from build123d import *

# Parameters (mm, degrees)
BOSS_EXTRUDE1_DEPTH = 30.5
SKETCH4_W           = 23.4
SKETCH4_H           = 13
CUT_EXTRUDE2_DEPTH  = 25
CUT_EXTRUDE4_DEPTH  = 11.5
SKETCH7_W           = 31
SKETCH7_H           = 1.7
BOSS_EXTRUDE3_DEPTH = 6
BOSS_EXTRUDE4_DEPTH = 6
LPATTERN1_COUNT     = 10
LPATTERN1_PITCH     = 3.1
SKETCH11_W          = 12
SKETCH11_H          = 4.5
BOSS_EXTRUDE5_DEPTH = 3
FILLET1_R           = 2
FILLET2_R           = 2
FILLET5_R           = 3
SKETCH12_W          = 3.5
SKETCH12_H          = 3.5
CUT_EXTRUDE5_DEPTH  = 12
FILLET6_R           = 1.5


with BuildPart() as part:
    # Sketch1 → Boss-Extrude1 (new body)
    with BuildSketch(Plane.XY):
        Polygon((0, 0), (0, -30), (12, -30), (12, -20), (5, 0), align=None)
    extrude(amount=-BOSS_EXTRUDE1_DEPTH)

    # Sketch4 → Cut-Extrude2 (cut)
    with BuildSketch(Plane.ZY):
        with Locations((-14.5, -25.899949695)):
            Rectangle(SKETCH4_W, SKETCH4_H)
    extrude(amount=-CUT_EXTRUDE2_DEPTH, mode=Mode.SUBTRACT)

    # Sketch6 → Cut-Extrude4 (cut, symmetric)
    with BuildSketch(Plane.XY.offset(-15.25)):
        Polygon((5, 0), (5, -14), (9.9, -14), align=None)
    extrude(amount=CUT_EXTRUDE4_DEPTH, both=True, mode=Mode.SUBTRACT)

    # Sketch7 → Boss-Extrude3 (add)
    with BuildSketch(Plane(origin=(0, -28, 0), x_dir=(1, 0, 0), z_dir=(0, 1, 0))):
        with Locations((-4.2231607, 25.4)):
            Rectangle(SKETCH7_W, SKETCH7_H)
    extrude(amount=BOSS_EXTRUDE3_DEPTH)

    # Sketch10 → Boss-Extrude4 (add)
    with BuildSketch(Plane(origin=(0, -28, 0), x_dir=(1, 0, 0), z_dir=(0, 1, 0))):
        with BuildLine():
            Line((9.930277247, 22.163714857), (9.488014181, 22.163714857))
            ThreePointArc((9.488014181, 22.163714857), (9.122148109, 23.010204326), (9.120849309, 23.932376064))
            ThreePointArc((9.120849309, 23.932376064), (8.970587763, 24.244009331), (8.809145714, 24.55))
            Line((8.809145714, 24.55), (10.609145714, 24.55))
            ThreePointArc((10.609145714, 24.55), (10.447703664, 24.244009331), (10.297442118, 23.932376064))
            ThreePointArc((10.297442118, 23.932376064), (10.296143319, 23.010204326), (9.930277247, 22.163714857))
        make_face()
    boss_extrude4 = extrude(amount=BOSS_EXTRUDE4_DEPTH)

    # LPattern1: Boss-Extrude4 ×10
    with Locations(*[(-i * LPATTERN1_PITCH, 0, 0) for i in range(1, LPATTERN1_COUNT)]):
        add(boss_extrude4)

    # Sketch11 → Boss-Extrude5 (add)
    with BuildSketch(Plane(origin=(0, 0, -30.5), x_dir=(-1, 0, 0), z_dir=(0, 0, -1))):
        with Locations((-6, -27.75)):
            Rectangle(SKETCH11_W, SKETCH11_H)
    boss_extrude5 = extrude(amount=BOSS_EXTRUDE5_DEPTH)

    # Fillet1
    fillet1_edges = [part.edges().sort_by_distance(p)[0] for p in [
        (6, -25.5, -33.5),
    ]]
    fillet(fillet1_edges, radius=FILLET1_R)

    # Mirror1: Boss-Extrude5 across plane
    add(boss_extrude5.mirror(Plane.XY.offset(-15.25)))

    # Fillet2
    fillet2_edges = [part.edges().sort_by_distance(p)[0] for p in [
        (6, -25.5, 3),
    ]]
    fillet(fillet2_edges, radius=FILLET2_R)

    # Fillet5
    fillet5_edges = [part.edges().sort_by_distance(p)[0] for p in [
        (5, -14, -15.25),
        (5.894991197, -19.399949695, -2.8),
    ]]
    fillet(fillet5_edges, radius=FILLET5_R)

    # Sketch12 → Cut-Extrude5 (cut)
    with BuildSketch(Plane.ZY):
        with Locations((-30.65, -28.814354386)):
            Rectangle(SKETCH12_W, SKETCH12_H)
        with Locations((0.15, -28.814354386)):
            Rectangle(SKETCH12_W, SKETCH12_H)
    extrude(amount=-CUT_EXTRUDE5_DEPTH, mode=Mode.SUBTRACT)

    # Fillet6
    fillet6_edges = [part.edges().sort_by_distance(p)[0] for p in [
        (6, -27.064354386, -28.9),
        (6, -27.064354386, -32.4),
        (6, -27.064354386, -1.6),
        (6, -27.064354386, 1.9),
    ]]
    fillet(fillet6_edges, radius=FILLET6_R)


solid = part.part
Could you check a few things on this model? Use its own coordinates, in mm. A direction names the side the tool comes from. Give positions to 0.01 mm unless a question says otherwise; leave off trailing zeros. Order: outer loops, then holes, each group sorted by start corner. A loop starts at its lowest first (then second) coordinate and runs counter-clockwise, first axis right, second up. Notation, with made-up numbers: M -12.75,71.5 L 26.25,71.5 A16 ccw 26.25,99.5 Z; hole C 83,-37 d3. An arc over 180 degrees is marked long. One line per question, with ' | ' between items.
1. I want a section at A-A (y = -3). List the corners of the cut face in (x, z) for me.
Results:
outline: M 0,-30.5 L 6.05,-30.5 L 6.05,-26.75 L 5,-26.75 L 5,-3.75 L 6.05,-3.75 L 6.05,0 L 0,0 Z
2. For faces 1 (the face through (2.925, -25.042, -22.997)), 2 (the face through (6, -29, 1.9)), 3 (the face through (5.9, -13.14, -15.09)), 4 (the face through (-7, -25, -24.55)), which set-ups out of +Z, -Z, +X, -X, +Y, -Y let a thin tool reach every point of the face, with its end or its side?
Results:
face 1: -Y | face 2: +X, -X, -Y | face 3: +X, +Y | face 4: +Z, +Y, -Y
3. We'd pull the mould along Z, two halves only. Please class faces 5 (the face through (6, -30, -33)), 6 (the face through (6, -19.4, -16)), 7 (the face through (-10, -25, -26.25)): +Z half, -Z half, draft (parallel to the pull), parting line (faces both ways), or undercut.
Results:
face 5: draft | face 6: undercut | face 7: -Z half
4. If I drill on line 1 (X direction, y = -2, z = -26); line 2 (Y direction, x = 4, z = -9); line 3 (Z direction, x = -10.5, y = -24.5), over which ranges is the centre line in solid material (lowest first)?
Results:
line 1: 0 to 5 | line 2: -19.4 to 0 | line 3: -26.25 to -24.55
5. I want a section at C-C (z = -8.5). List the corners of the cut face in (x, y) for me.
Results:
outline: M 0,-19.4 L 11.79,-19.4 L 9.9,-14 L 8,-14 A3 cw 5,-11 L 5,0 L 0,0 Z
6. I want a section at D-D (y = -21). List the corners of the cut face in (x, z) for me, and give its area (3 significant figures).
Results:
outline: M 0,-30.5 L 12,-30.5 L 12,-26.2 L 0,-26.2 Z; M 0,-3.15 L 12,-3.15 L 12,0 L 0,0 Z | area: 89.4 mm²
7. I'm going to push flat-ended pins straight in: pin 1 (9.5 mm diameter, centred on x = 7.5, y = -14, fed in from -Z); pin 2 (1.5 mm diameter, centred on y = -23.5, z = -23.5, fed in from -X); pin 3 (0.6 mm diameter, centred on x = -11, y = -24, fed in from +Z); pin 4 (2 mm diameter, centred on x = 2.5, z = -23.5, fed in from +Y). Where does each tip first touch, or does it pass through?
Results:
pin 1: z = -30.5 | pin 2: x = -18.93 | pin 3: z = -24.15 | pin 4: y = 0
